Part model, mm, in its own coordinate system. A direction names the side the tool comes from. Round coordinates to 2 decimals unless told otherwise and drop trailing zeros. Order: outer loops, then holes, each group sorted by start corner. A loop starts at its lowest first (then second) coordinate and runs counter-clockwise, first axis right, second up. Notation, with made-up numbers: (72, 78) - (102, 78) arc R21 cw to (102, 83) - close; hole circle Ø1 at (34.5, -40). An arc over 180 degrees is marked (long way). Answer as a JSON object with one key per item and string values.
```python
from build123d import *

# Parameters (mm, degrees)
SALIENTE_EXTRUIR1_DEPTH      = 6.35
TALADRO_DE_MARGEN_PARA_M41_D = 4.5
REDONDEO1_R                  = 5
TALADRO_DE_MARGEN_PARA_M42_D = 4.5


with BuildPart() as part:
    # Croquis1 → Saliente-Extruir1 (new body)
    with BuildSketch(Plane(origin=(0, 0, 0), x_dir=(0, 0, -1), z_dir=(1, 0, 0))):
        Polygon((-22.5, 85), (-22.5, 55), (22.5, 55), (22.5, 85), (37.5, 85), (37.5, 35), (37.5, -35), (37.5, -85), (22.5, -85), (22.5, -55), (-22.5, -55), (-22.5, -85), (-37.5, -85), (-37.5, -35), (-37.5, 35), (-37.5, 85), align=None)
    extrude(amount=SALIENTE_EXTRUIR1_DEPTH)

    # Taladro de margen para M41 (through all)
    with Locations(Plane.ZY):
        with Locations((30, 68), (30, 80), (-30, 68), (-30, 80), (30, -80), (30, -68), (-30, -80), (-30, -68)):
            Hole(TALADRO_DE_MARGEN_PARA_M41_D / 2)

    # Redondeo1
    redondeo1_edges = [part.edges().sort_by_distance(p)[0] for p in [
        (3.175, 85, 22.5),
        (3.175, 85, -22.5),
        (3.175, 85, -37.5),
        (3.175, -85, -37.5),
        (3.175, -85, -22.5),
        (3.175, -85, 22.5),
        (3.175, -85, 37.5),
        (3.175, 85, 37.5),
    ]]
    fillet(redondeo1_edges, radius=REDONDEO1_R)

    # Taladro de margen para M42 (through all)
    with Locations(Plane(origin=(6.35, 0, 0), x_dir=(0, 0, -1), z_dir=(1, 0, 0))):
        with Locations((-17.5, -10), (17.5, -10), (17.5, -22), (-17.5, -22)):
            Hole(TALADRO_DE_MARGEN_PARA_M42_D / 2)


solid = part.part
```
Item 1: Cut at D-D (x = 5). State how many separate pieces and enclosed holes the cut face has, plus the area to 3 significant figures.
Taken from the geometry:
{"separate pieces": "1", "enclosed holes": "12", "area": "9,820 mm2"}
Item 2: Cut at B-B (z = 17.5). Write the cut outline in (x, y), plus the area to 3 significant figures.
Taken from the geometry:
{"outline": "(0, -55) - (6.35, -55) - (6.35, -24.25) - (0, -24.25) - close; (0, -19.75) - (6.35, -19.75) - (6.35, -12.25) - (0, -12.25) - close; (0, -7.75) - (6.35, -7.75) - (6.35, 55) - (0, 55) - close", "area": "641 mm2"}
Item 3: Probe L1, parallel to Y at x = 2, z = 17.5; L2, parallel to Z at x = 4, y = -70.5; L3, parallel to Z at x = 2.75, y = -23. List the from-to ranges inside material, lowest first. Write a range as from..to.
Taken from the geometry:
{"L1": "-55..-24.25, -19.75..-12.25, -7.75..55", "L2": "-37.5..-22.5, 22.5..37.5", "L3": "-37.5..-19.52, -15.48..15.48, 19.52..37.5"}
Item 4: Drop flat-ended pins along their axis: P1, Ø5, axis at y = -80, z = -30, coming from the +X side; P2, Ø1.5, axis at x = 4, z = 7, coming from the +Y side. Give the stop position or say it passes through.
Taken from the geometry:
{"P1": "x = 6.35", "P2": "y = 55"}
Item 5: Two-plate mould, pull along Z, no slides. Class faces 1 (the cylindrical face through (3.219, -70.196, -29.512)), 2 (the cylindrical face through (3.22, 83.57, -36)), 3 (the flat face through (3, -85, 30)), 4 (the cylindrical face through (3.131, -8.103, -16.29)): pulls with the +Z half, pulls with the -Z half, needs draft (parallel to the pull), parting line crosses it, or undercut.
Taken from the geometry:
{"face 1": "undercut", "face 2": "pulls with the -Z half", "face 3": "needs draft", "face 4": "undercut"}
Item 6: Cut at C-C (y = -22). Write the cut outline in (x, z).
Taken from the geometry:
{"outline": "(0, -37.5) - (6.35, -37.5) - (6.35, -19.75) - (0, -19.75) - close; (0, -15.25) - (6.35, -15.25) - (6.35, 15.25) - (0, 15.25) - close; (0, 19.75) - (6.35, 19.75) - (6.35, 37.5) - (0, 37.5) - close"}
Item 7: Cut at A-A (y = -63). Write the cut outline in (x, z), plus the area to 4 significant figures.
Taken from the geometry:
{"outline": "(0, -37.5) - (6.35, -37.5) - (6.35, -22.5) - (0, -22.5) - close; (0, 22.5) - (6.35, 22.5) - (6.35, 37.5) - (0, 37.5) - close", "area": "190.5 mm2"}
Item 8: Tool access for faces 5 (the flat face through (3, 67, -22.5)), 6 (the cylindrical face through (3.219, -82.196, -29.512)), 7 (the flat face through (3, -55, 0)): list every direction of +Z, -Z, +X, -X, +Y, -Y with a clear straight run to the whole face (end or side of a thin tool).
Taken from the geometry:
{"face 5": "+X, -X, +Y", "face 6": "+X, -X", "face 7": "+X, -X, -Y"}
